The listing builds one solid part. Answer for the finished solid, in the listing's coordinates (mm). Give positions to 0.01 mm unless a question says otherwise; leave off trailing zeros. Write each loop counter-clockwise with the first axis right and the second up, starting at its lowest first coordinate (ties: lowest second). Pieces come first, ordered by that corner, then holes. Notation, with made-up numbers: (49.25, 68.5) -> (66.25, 68.5) arc R28 ccw to (66.25, 100.5) -> close; hole circle Ø9 at (-25, -23). An arc over 180 degrees is marked (long way). One line per question, with ' | ' between items.
from build123d import *

# Parameters (mm, degrees)
F2_R = 4.99999
F3_R = 5


# Not quite as in the source:
# - a fillet or chamfer is up to 0.001 mm smaller than in the source, because OpenCascade refuses the exact size


with BuildPart() as f1:
    # F0 (on Front) → F1 (revolve)
    with BuildSketch(Plane.XZ):
        with BuildLine():
            Line((0, 120), (0, 0))
            Line((0, 0), (60, 0))
            Line((60, 0), (60, 5))
            Line((60, 5), (20, 5))
            Line((20, 5), (60, 60))
            ThreePointArc((60, 60), (42.4264068712, 102.4264068712), (0, 120))
        make_face()
    revolve(axis=Axis((0, 0, 60), (0, 0, -1)))

    # F2 (radius 5 in the source; OpenCascade refuses exactly that, so slightly less here)
    f2_edges = [f1.edges().sort_by_distance(p)[0] for p in [
        (-60, 0, 5),
        (-20, 0, 5),
    ]]
    fillet(f2_edges, radius=F2_R)

    # F3
    f3_edges = [f1.edges().sort_by_distance(p)[0] for p in [
        (-60, 0, 60),
    ]]
    fillet(f3_edges, radius=F3_R)


solid = f1.part
Item 1: Flat-ended cylindrical pins translate along their axes: pin 1 (6 mm diameter, centred on y = 26.5, z = 37.5, fed in from -X); pin 2 (1.5 mm diameter, centred on x = -37.5, z = 98.5, fed in from -Y); pin 3 (10 mm diameter, centred on x = 44.5, y = 20.5, fed in from +Z). Find the tip coordinate at first contact, or state that the pin passes through.
Answers below:
pin 1: x = -38.07 | pin 2: y = -28.13 | pin 3: z = 100.8
Item 2: Determine the mould class of faces 1 (the face through (1, -1, 0)), 2 (the face through (25.73, 10.67, 15.8)) for opening direction Z: pulls with the +Z half, pulls with the -Z half, needs draft (parallel to the pull), parting line crosses it, or undercut.
Answers below:
face 1: pulls with the -Z half | face 2: undercut
Item 3: Consider line 1 (Z direction, x = 26, y = 0.5); line 2 (Z direction, x = 20.5, y = -26); line 3 (Y direction, x = 22, z = 62.5). Determine where each line is inside the solid, lowest interval first. Write a range as [from, to].
Answers below:
line 1: [0, 6.77], [13.26, 114.07] | line 2: [0, 5], [23.03, 110.04] | line 3: [-55.77, 55.77]
Item 4: Find section A-A (z = 22.5). Write down the section's boundary in (x, y).
Answers below:
outline: circle Ø65.45 at (0, 0)
Item 5: Find section B-B (z = 34.5). Write down the section's boundary in (x, y).
Answers below:
outline: circle Ø82.91 at (0, 0)
